Source: CAD feature listing. Evaluate the final solid. Frame: model axes, mm. A direction names the side the tool comes from. Coordinates: 2 decimals unless noted, no trailing zeros. Write each loop counter-clockwise with the first axis right and the second up, starting at its lowest first coordinate (ties: lowest second). Pieces come first, ordered by that corner, then holes. Notation, with made-up numbers: (84.5, -30.5) - (107.5, -30.5) arc R21 cw to (107.5, -22.5) - close; hole circle Ø1 at (-10.5, 51). An arc over 180 degrees is marked (long way). One line per item, written item: value.
from build123d import *

# Parameters (mm, degrees)
SKETCH1_R           = 19
SKETCH1_R_2         = 5.08
BOSS_EXTRUDE1_DEPTH = 2.032
CUT_EXTRUDE1_DEPTH  = 27.946781329
CIRPATTERN1_COUNT   = 2
CIRPATTERN1_ANGLE   = 90
SKETCH3_W           = 5.08
SKETCH3_H           = 5.08
BOSS_EXTRUDE2_DEPTH = 2.54
CIRPATTERN2_COUNT   = 6


with BuildPart() as part:
    # Sketch1 → Boss-Extrude1 (new body)
    with BuildSketch(Plane(origin=(0, 0, 0), x_dir=(1, 0, 0), z_dir=(0, 1, 0))):
        with Locations(Location((0, 0, 0), (0, 0, 270))):
            Circle(SKETCH1_R)
        with Locations(Location((0, 0, 0), (0, 0, 270))):
            Circle(SKETCH1_R_2, mode=Mode.SUBTRACT)
    extrude(amount=BOSS_EXTRUDE1_DEPTH)

    # Sketch2 → Cut-Extrude1 (cut, through all)
    with BuildSketch(Plane(origin=(0, 2.032, 0), x_dir=(1, 0, 0), z_dir=(0, 1, 0))):
        with BuildLine():
            Line((-4.678437239, 18.415), (4.678437239, 18.415))
            ThreePointArc((4.678437239, 18.415), (0, 19), (-4.678437239, 18.415))
        make_face()
        with BuildLine():
            Line((-4.678437239, -18.415), (4.678437239, -18.415))
            ThreePointArc((4.678437239, -18.415), (0, -19), (-4.678437239, -18.415))
        make_face()
    cut_extrude1 = extrude(amount=-CUT_EXTRUDE1_DEPTH, mode=Mode.SUBTRACT)

    # CirPattern1: Cut-Extrude1 ×2 about axis
    cirpattern1_axis = Axis((0, 2.032, 0), (0, -1, 0))
    for i in range(1, CIRPATTERN1_COUNT):
        add(cut_extrude1.rotate(cirpattern1_axis, i * CIRPATTERN1_ANGLE / (CIRPATTERN1_COUNT - 1)), mode=Mode.SUBTRACT)

    # Sketch3 → Boss-Extrude2 (add)
    with BuildSketch(Plane(origin=(0, 2.032, 0), x_dir=(1, 0, 0), z_dir=(0, 1, 0))):
        with Locations((0, 14.605)):
            Rectangle(SKETCH3_W, SKETCH3_H)
    boss_extrude2 = extrude(amount=BOSS_EXTRUDE2_DEPTH)

    # CirPattern2: Boss-Extrude2 ×6 about axis
    cirpattern2_axis = Axis((0, 0, 0), (0, 1, 0))
    for i in range(1, CIRPATTERN2_COUNT):
        add(boss_extrude2.rotate(cirpattern2_axis, i * 360 / CIRPATTERN2_COUNT))


solid = part.part
1) Section query D-D on x = -14. Output: boundary loops of the cut face in (y, z).
Values found:
outline: (0, -12.85) - (2.03, -12.85) - (2.03, -10.04) - (4.57, -10.04) - (4.57, -5.15) - (2.03, -5.15) - (2.03, 5.15) - (4.57, 5.15) - (4.57, 10.04) - (2.03, 10.04) - (2.03, 12.85) - (0, 12.85) - close
2) Contact query for flat-ended pins moving along their axis: P1, Ø1, axis at x = 14, y = 3, coming from the -Z side; P2, Ø1.5, axis at y = 3.5, z = -8, coming from the -X side; P3, Ø1.5, axis at y = 0.5, z = 7.5, coming from the -X side; P4, Ø8, axis at x = 0, z = 0, coming from the +Y side. Output: stop coordinate, or through.
Values found:
P1: z = -10.77
P2: x = -15.61
P3: x = -17.76
P4: through
3) Section query C-C on x = 0. Output: boundary loops of the cut face in (y, z) (3 decimals), then the cut area to 3 significant figures.
Values found:
outline: (0, -18.415) - (2.032, -18.415) - (2.032, -17.145) - (4.572, -17.145) - (4.572, -12.065) - (2.032, -12.065) - (2.032, -5.08) - (0, -5.08) - close; (0, 5.08) - (2.032, 5.08) - (2.032, 12.065) - (4.572, 12.065) - (4.572, 17.145) - (2.032, 17.145) - (2.032, 18.415) - (0, 18.415) - close
area: 80.0 mm2
4) Section query A-A on y = 3.1. Output: boundary loops of the cut face in (x, z) (3 decimals), then the cut area to 3 significant figures.
Values found:
outline: (-16.118, -6.373) - (-13.578, -10.772) - (-9.179, -8.232) - (-11.719, -3.833) - close; (-16.118, 6.373) - (-11.719, 3.833) - (-9.179, 8.232) - (-13.578, 10.772) - close; (-2.54, -17.145) - (2.54, -17.145) - (2.54, -12.065) - (-2.54, -12.065) - close; (-2.54, 12.065) - (2.54, 12.065) - (2.54, 17.145) - (-2.54, 17.145) - close; (9.179, -8.232) - (13.578, -10.772) - (16.118, -6.373) - (11.719, -3.833) - close; (9.179, 8.232) - (11.719, 3.833) - (16.118, 6.373) - (13.578, 10.772) - close
area: 155 mm2
5) Draft query along X for faces 4 (the cylindrical face through (-13.33, 1, -13.54)), 5 (the cylindrical face through (5.037, 1.002, -0.661)), 6 (the flat face through (10.466, 3.284, 6.002)), 7 (the flat face through (4, 0, 4)). Return one class per face: released by +X, released by -X, zero draft, split by the parting line, or undercut.
Values found:
face 4: released by -X
face 5: undercut
face 6: undercut
face 7: zero draft
6) Material intervals for line 1 (X direction, y = 1.2, z = 0) (3 decimals); line 2 (Z direction, x = -0.5, y = 3.75) (3 decimals); line 3 (X direction, y = 4.35, z = 14), sorted ascending.
Values found:
line 1: -18.415 to -5.08, 5.08 to 18.415
line 2: -17.145 to -12.065, 12.065 to 17.145
line 3: -2.54 to 2.54
7) Reachability of faces 1 (the flat face through (-10.431, 3.284, 6.063)), 2 (the flat face through (2.54, 3, 15)), 3 (the flat face through (-2.54, 3, 15)) from +Z, -Z, +X, -X, +Y, -Y: full face, straight path, thin tool, end or side. Return the list, or none.
Values found:
face 1: +Y
face 2: +Z, -Z, +X, +Y
face 3: +Z, -Z, -X, +Y
8) Section query B-B on z = 0. Output: boundary loops of the cut face in (x, y) (3 decimals).
Values found:
outline: (-18.415, 0) - (-5.08, 0) - (-5.08, 2.032) - (-18.415, 2.032) - close; (5.08, 0) - (18.415, 0) - (18.415, 2.032) - (5.08, 2.032) - close
